from build123d import *

# Parameters (mm, degrees)
SKETCH_1_W                   = 120
SKETCH_1_H                   = 120
SKETCH_1_W_2                 = 28
SKETCH_1_H_2                 = 50
SM_BASE_FLANGE_1_DEPTH       = 4
SM_START                     = -5
SM_EDGE_FLANGE_1_DEPTH       = 10
SM_EDGE_FLANGE_1_2_OUTLINE_W = 26
SM_EDGE_FLANGE_1_2_OUTLINE_H = 4
SM_EDGE_FLANGE_1_2_DEPTH     = 1.41096
SM_START_2                   = 5
SM_EDGE_FLANGE_1_3_OUTLINE_W = 26
SM_EDGE_FLANGE_1_3_OUTLINE_H = 4
SM_EDGE_FLANGE_1_3_DEPTH     = 20
SM_START_3                   = -13
SM_EDGE_FLANGE_1_4_DEPTH     = 26
SM_EDGE_FLANGE_1_5_DEPTH     = 26
CUT_EXTRUDE_1_DEPTH          = 89.459030065
CUT_EXTRUDE_1_DEPTH_BACK     = 89.459030065
SKETCH_10_R                  = 4.05
SKETCH_12_W                  = 8.2
SKETCH_12_H                  = 8.2
CUT_EXTRUDE_3_DEPTH          = 4
FILLET_1_R                   = 10
SKETCH_11_R                  = 4
CUT_EXTRUDE_2_DEPTH          = 4
CUT_EXTRUDE_4_DEPTH          = 4
CUT_EXTRUDE_5_DEPTH          = 4
FILLET_2_R                   = 15


with BuildPart() as part:
    # Базовая кромка1: sheet metal written as solids
    # Sketch 1 → Базовая кромка1 (new body)
    with BuildSketch(Plane.XY):
        Rectangle(SKETCH_1_W, SKETCH_1_H)
        Rectangle(SKETCH_1_W_2, SKETCH_1_H_2, mode=Mode.SUBTRACT)
    extrude(amount=-SM_BASE_FLANGE_1_DEPTH)

    # Ребро-кромка1: read off the stored shape, not the designer's step
    # Ребро-кромка1 outline → Ребро-кромка1 (cut)
    with BuildSketch(Plane.XY.offset(SM_START)):
        with BuildLine():
            ThreePointArc((-13, 34.1), (-13.5, 34.6), (-14, 34.1))
            Line((-14, 34.1), (-14, 25))
            Line((-14, 25), (-13, 25))
            Line((-13, 25), (-13, 34.1))
        make_face()
        with BuildLine():
            Line((-13, -25), (-14, -25))
            Line((-14, -25), (-14, -34.1))
            ThreePointArc((-14, -34.1), (-13.5, -34.6), (-13, -34.1))
            Line((-13, -34.1), (-13, -25))
        make_face()
        with BuildLine():
            Line((13, 34.1), (13, 25))
            Line((13, 25), (14, 25))
            Line((14, 25), (14, 34.1))
            ThreePointArc((14, 34.1), (13.5, 34.6), (13, 34.1))
        make_face()
        with BuildLine():
            Line((14, -25), (13, -25))
            Line((13, -25), (13, -34.1))
            ThreePointArc((13, -34.1), (13.5, -34.6), (14, -34.1))
            Line((14, -34.1), (14, -25))
        make_face()
    extrude(amount=SM_EDGE_FLANGE_1_DEPTH, mode=Mode.SUBTRACT)

    # Sm Edge Flange 1 2 outline → Sm Edge Flange 1 2 (cut)
    with BuildSketch(Plane.XY.offset(SM_START)):
        with Locations((0, 27)):
            Rectangle(SM_EDGE_FLANGE_1_2_OUTLINE_W, SM_EDGE_FLANGE_1_2_OUTLINE_H)
        with Locations((0, -27)):
            Rectangle(SM_EDGE_FLANGE_1_2_OUTLINE_W, SM_EDGE_FLANGE_1_2_OUTLINE_H)
    extrude(amount=SM_EDGE_FLANGE_1_2_DEPTH, mode=Mode.SUBTRACT)

    # Sm Edge Flange 1 4 outline → Sm Edge Flange 1 4 (cut)
    with BuildSketch(Plane.YZ.offset(SM_START_3)):
        with BuildLine():
            ThreePointArc((34, -4), (29.757359313, -2.937253933), (26.516685226, 0))
            Line((26.516685226, 0), (25, 0))
            Line((25, 0), (25, -3.58904))
            Line((25, -3.58904), (29, -3.58904))
            Line((29, -3.58904), (29, -4))
            Line((29, -4), (34, -4))
        make_face()
        with BuildLine():
            Line((-25, -3.58904), (-25, 0))
            Line((-25, 0), (-26.516685226, 0))
            ThreePointArc((-26.516685226, 0), (-29.757359313, -2.937253933), (-34, -4))
            Line((-34, -4), (-29, -4))
            Line((-29, -4), (-29, -3.58904))
            Line((-29, -3.58904), (-25, -3.58904))
        make_face()
    extrude(amount=SM_EDGE_FLANGE_1_4_DEPTH, mode=Mode.SUBTRACT)



with BuildPart() as body_2:
    # Sm Edge Flange 1 3 outline → Sm Edge Flange 1 3 (new body)
    with BuildSketch(Plane.XY.offset(SM_START_2)):
        with Locations((0, 27)):
            Rectangle(SM_EDGE_FLANGE_1_3_OUTLINE_W, SM_EDGE_FLANGE_1_3_OUTLINE_H)
        with Locations((0, -27)):
            Rectangle(SM_EDGE_FLANGE_1_3_OUTLINE_W, SM_EDGE_FLANGE_1_3_OUTLINE_H)
    extrude(amount=SM_EDGE_FLANGE_1_3_DEPTH)


with BuildPart() as part_1:
    add(part.part)

    add(body_2.part)  # Sm Edge Flange 1 5 merges body 2
    # Sm Edge Flange 1 5 outline → Sm Edge Flange 1 5 (add)
    with BuildSketch(Plane.YZ.offset(SM_START_3)):
        with BuildLine():
            Line((29, 5), (25, 5))
            ThreePointArc((25, 5), (25.38751392, 2.38751392), (26.516685226, 0))
            Line((26.516685226, 0), (34, 0))
            ThreePointArc((34, 0), (30.464466094, 1.464466094), (29, 5))
        make_face()
        with BuildLine():
            Line((-34, 0), (-26.516685226, 0))
            ThreePointArc((-26.516685226, 0), (-25.38751392, 2.38751392), (-25, 5))
            Line((-25, 5), (-29, 5))
            ThreePointArc((-29, 5), (-30.464466094, 1.464466094), (-34, 0))
        make_face()
    extrude(amount=SM_EDGE_FLANGE_1_5_DEPTH)

    # Эскиз10 → Вырез-Вытянуть1 (cut, two sides: drawn at the far end of the back side and taken through both)
    with BuildSketch(Plane(origin=(0, 0, 0), x_dir=(1, 0, 0), z_dir=(0, 1, 0)).offset(-CUT_EXTRUDE_1_DEPTH_BACK)):
        with Locations(Location((0, -17, 0), (0, 0, 90))):
            Circle(SKETCH_10_R)
    extrude(amount=CUT_EXTRUDE_1_DEPTH + CUT_EXTRUDE_1_DEPTH_BACK, mode=Mode.SUBTRACT)

    # Эскиз12 → Вырез-Вытянуть3 (cut)
    with BuildSketch(Plane(origin=(0, 29, 0), x_dir=(1, 0, 0), z_dir=(0, 1, 0))):
        with Locations((0, -17)):
            Rectangle(SKETCH_12_W, SKETCH_12_H)
    extrude(amount=-CUT_EXTRUDE_3_DEPTH, mode=Mode.SUBTRACT)

    # Скругление1
    fillet_1_edges = [part_1.edges().sort_by_distance(p)[0] for p in [
        (13, -27, 25),
        (-13, -27, 25),
        (-60, 60, -2),
        (60, 60, -2),
        (60, -60, -2),
        (-60, -60, -2),
        (-13, 27, 25),
        (13, 27, 25),
    ]]
    fillet(fillet_1_edges, radius=FILLET_1_R)

    # Эскиз11 → Вырез-Вытянуть2 (cut)
    with BuildSketch(Plane.XY):
        with Locations((-51, 51)):
            Circle(SKETCH_11_R)
        with Locations((51, 51)):
            Circle(SKETCH_11_R)
        with Locations((-51, -51)):
            Circle(SKETCH_11_R)
        with Locations((51, -51)):
            Circle(SKETCH_11_R)
    extrude(amount=-CUT_EXTRUDE_2_DEPTH, mode=Mode.SUBTRACT)

    # Эскиз13 → Вырез-Вытянуть4 (cut)
    with BuildSketch(Plane.XY):
        with BuildLine():
            Line((-48.171572875, 53.828427125), (-44.636038969, 50.292893219))
            ThreePointArc((-44.636038969, 50.292893219), (-44.636038969, 44.636038969), (-50.292893219, 44.636038969))
            Line((-50.292893219, 44.636038969), (-53.828427125, 48.171572875))
            ThreePointArc((-53.828427125, 48.171572875), (-53.828427125, 53.828427125), (-48.171572875, 53.828427125))
        make_face()
        with BuildLine():
            Line((53.828427125, 48.171572875), (50.292893219, 44.636038969))
            ThreePointArc((50.292893219, 44.636038969), (44.636038969, 44.636038969), (44.636038969, 50.292893219))
            Line((44.636038969, 50.292893219), (48.171572875, 53.828427125))
            ThreePointArc((48.171572875, 53.828427125), (53.828427125, 53.828427125), (53.828427125, 48.171572875))
        make_face()
        with BuildLine():
            Line((-53.828427125, -48.171572875), (-50.292893219, -44.636038969))
            ThreePointArc((-50.292893219, -44.636038969), (-44.636038969, -44.636038969), (-44.636038969, -50.292893219))
            Line((-44.636038969, -50.292893219), (-48.171572875, -53.828427125))
            ThreePointArc((-48.171572875, -53.828427125), (-53.828427125, -53.828427125), (-53.828427125, -48.171572875))
        make_face()
        with BuildLine():
            Line((48.171572875, -53.828427125), (44.636038969, -50.292893219))
            ThreePointArc((44.636038969, -50.292893219), (44.636038969, -44.636038969), (50.292893219, -44.636038969))
            Line((50.292893219, -44.636038969), (53.828427125, -48.171572875))
            ThreePointArc((53.828427125, -48.171572875), (53.828427125, -53.828427125), (48.171572875, -53.828427125))
        make_face()
    extrude(amount=-CUT_EXTRUDE_4_DEPTH, mode=Mode.SUBTRACT)

    # Эскиз14 → Вырез-Вытянуть5 (cut)
    with BuildSketch(Plane.XY):
        with BuildLine():
            Line((-60, 40), (-60, -40))
            ThreePointArc((-60, -40), (-40, 0), (-60, 40))
        make_face()
        with BuildLine():
            Line((60, 40), (60, -40))
            ThreePointArc((60, -40), (40, 0), (60, 40))
        make_face()
        with BuildLine():
            Line((-40, 60), (40, 60))
            ThreePointArc((40, 60), (0, 51.651513899), (-40, 60))
        make_face()
        with BuildLine():
            Line((-40, -60), (40, -60))
            ThreePointArc((40, -60), (0, -51.651513899), (-40, -60))
        make_face()
    extrude(amount=-CUT_EXTRUDE_5_DEPTH, mode=Mode.SUBTRACT)

    # Скругление2
    fillet_2_edges = [part_1.edges().sort_by_distance(p)[0] for p in [
        (40, 60, -2),
        (-40, 60, -2),
        (60, -40, -2),
        (60, 40, -2),
        (-40, -60, -2),
        (40, -60, -2),
        (-60, 40, -2),
        (-60, -40, -2),
    ]]
    fillet(fillet_2_edges, radius=FILLET_2_R)


solid = part_1.part
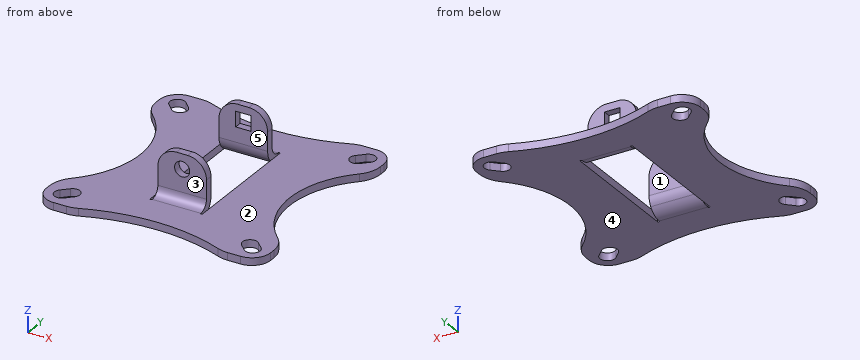
The model under review builds one solid part; all positions refer to its coordinate system, in mm. Face numbers are marked on the shaded views. A direction names the side the tool comes from. Coordinates: 2 decimals unless noted, no trailing zeros. Write each loop counter-clockwise with the first axis right and the second up, starting at its lowest first coordinate (ties: lowest second). Pieces come first, ordered by that corner, then holes. Notation, with made-up numbers: M 14,9.5 L 48,9.5 A29 ccw 48,37.5 Z; hole C 59.25,51.5 d6. An arc over 180 degrees is marked long. Put each result on its own line as item: value.
1) For the marked faces 4 and 5, list the 3-axis set-ups (+Z, -Z, +X, -X, +Y, -Y) from which the entire face can be reached by the end or side of a thin tool; tool diameter is ignored.
Computed:
face 4: -Z, +X, -X, +Y, -Y
face 5: +Z, -Z, +X, -X
2) Add section A-A on z = 11.5. Give the boundary of the cut face in (x, y).
Computed:
outline: M -13,-29 L 13,-29 L 13,-25 L -13,-25 Z; M -13,25 L 13,25 L 13,29 L -13,29 Z
3) Add section B-B on x = -6.5. Give the boundary of the cut face in (y, z), then the cut area to 3 significant figures.
Computed:
outline: M -51.86,-4 L -34,-4 A9 ccw -25,5 L -25,24.37 L -29,24.37 L -29,5 A5 cw -34,0 L -51.86,0 Z; M 25,5 A9 ccw 34,-4 L 51.86,-4 L 51.86,0 L 34,0 A5 cw 29,5 L 29,24.37 L 25,24.37 Z
area: 386 mm2
4) Add section C-C on y = 2. Give the boundary of the cut face in (x, z), then the cut area to 3 significant figures.
Computed:
outline: M -40.04,-4 L -14,-4 L -14,0 L -40.04,0 Z; M 14,-4 L 40.04,-4 L 40.04,0 L 14,0 Z
area: 208 mm2
5) Clearance check with flat-ended pins moving along their axes: pin 1 Ø2 at (x, z) = (-6, 20.5) entering from +Y; pin 2 Ø7.5 at (y, z) = (-29.5, 2) entering from +X; pin 3 Ø4.5 at (y, z) = (27.5, 16.5) entering from -X. State where each tip first meets the part, or that it passes through.
Computed:
pin 1: stops at y = 29
pin 2: stops at x = 52.15
pin 3: stops at x = -13
6) Draft analysis for pull direction Y (two halves, no side actions). For the marked faces 1, 2 and 3, state which applies: released by +Y, released by -Y, zero draft, split by the parting line, or undercut.
Computed:
face 1: undercut
face 2: zero draft
face 3: released by -Y
7) Wall thickness on probe 1 along Z at (x, y) = (-32, -33); probe 2 along X at (y, z) = (-26.2, 17); probe 3 along X at (y, z) = (11.5, -1): over which ranges is each line inside the solid? List them lowest first. Write a range as [from, to].
Computed:
probe 1: z = [-4, 0]
probe 2: x = [-12.8, -4.05], [4.05, 12.8]
probe 3: x = [-41.34, -14], [14, 41.34]
8) Add section D-D on z = 19.25. Give the boundary of the cut face in (x, y), then the cut area to 3 significant figures.
Computed:
outline: M -12.05,-29 L -3.37,-29 L -3.37,-25 L -12.05,-25 Z; M -12.05,25 L -4.1,25 L -4.1,29 L -12.05,29 Z; M 3.37,-29 L 12.05,-29 L 12.05,-25 L 3.37,-25 Z; M 4.1,25 L 12.05,25 L 12.05,29 L 4.1,29 Z
area: 133 mm2
